```python
from build123d import *

# Parameters (mm, degrees)
VACIADO1_START                    = -69.409306307
VACIADO1_OUTLINE_R                = 22.113173388
VACIADO1_DEPTH                    = 111.965075994
CROQUIS3_W                        = 3
CROQUIS3_H                        = 111.238505794
SALIENTE_EXTRUIR1_DEPTH           = 85
SALIENTE_EXTRUIR1_TAPER           = -0.018
SALIENTE_EXTRUIR1_OTHER_WAY_DEPTH = 2


# Read off the part's stored shape, not the designer's step: Vaciado1
with BuildPart() as part:
    # Croquis1 → Revolución1 (revolve)
    with BuildSketch(Plane.XY, mode=Mode.PRIVATE) as revoluci_n1_sk:
        Polygon((0, 52.555769687), (0, 46.993844398), (0, -69.409306307), (35.29141641, -69.409306307), (35.29141641, -64.244661396), (32.113173388, -64.244661396), (32.113173388, 46.993844398), (35.29141641, 46.993844398), (35.29141641, 52.555769687), align=None)
    revolve(revoluci_n1_sk.sketch.rotate(Axis((0, -77.4814163, 0), (0, 1, 0)), 90), axis=Axis((0, -77.4814163, 0), (0, 1, 0)))

    # Vaciado1 outline → Vaciado1 (cut)
    with BuildSketch(Plane(origin=(0, 0, 0), x_dir=(1, 0, 0), z_dir=(0, 1, 0)).offset(VACIADO1_START)):
        Circle(VACIADO1_OUTLINE_R)
    extrude(amount=VACIADO1_DEPTH, mode=Mode.SUBTRACT)

    # Croquis3 → Saliente-Extruir1 (add)
    with BuildSketch(Plane(origin=(35.21176327, 0, 0), x_dir=(1, 0, 0), z_dir=(0, 0, 1))):
        with Locations((0, -8.625408499)):
            Rectangle(CROQUIS3_W, CROQUIS3_H)
    extrude(amount=-SALIENTE_EXTRUIR1_DEPTH, taper=SALIENTE_EXTRUIR1_TAPER)

    # Croquis3 → Saliente-Extruir1 other way (add)
    with BuildSketch(Plane(origin=(35.21176327, 0, 0), x_dir=(1, 0, 0), z_dir=(0, 0, 1))):
        with Locations((0, -8.625408499)):
            Rectangle(CROQUIS3_W, CROQUIS3_H)
    extrude(amount=SALIENTE_EXTRUIR1_OTHER_WAY_DEPTH)


solid = part.part
```
Could you check a few things on this model? Use its own coordinates, in mm. A direction names the side the tool comes from. Give positions to 0.01 mm unless a question says otherwise; leave off trailing zeros. Order: outer loops, then holes, each group sorted by start corner. A loop starts at its lowest first (then second) coordinate and runs counter-clockwise, first axis right, second up.
Q1. I'm going to push flat-ended pins straight in: P1, Ø8, axis at x = 27, z = -30.5, coming from the +Y side; P2, Ø12, axis at x = -4, y = 37.5, coming from the +Z side; P3, Ø1.2, axis at x = 36.5, z = 1, coming from the -Y side; P4, Ø13.5, axis at x = -2, z = 2.5, coming from the -Y side. Where does each tip first touch, or does it pass through?
Q2. Suppose I cut it at D-D, the plane x = -25. Write out the boundary of the cut face in (y, z), and give its area (3 significant figures).
Q3. Suppose I cut it at B-B, the plane x = 0. Write out the boundary of the cut face in (y, z).
Q4. Suppose I cut it at A-A, the plane y = 37. Count the separate pieces of the cut face and the enclosed holes in it, and give its area (3 significant figures).
Q5. If I drill on line 1 along X through (y, z) = (-19, 0); line 2 along Y through (x, z) = (-25, 22); line 3 along X through (y, z) = (11.5, -66), over which ranges is the centre line in solid material (lowest first)?
Q6. For faces 1 (the cylindrical face through (11.888, -14.211, -18.646)), 2 (the flat face through (-32, -64.245, -8)), 3 (the flat face through (35, -8, 2)), 4 (the flat face through (23, -69.409, 0)), which set-ups out of +Z, -Z, +X, -X, +Y, -Y let a thin tool reach every point of the face, with its end or its side?
Q7. We'd pull the mould along Z, two halves only. Please class faces 5 (the flat face through (0, 52.556, 0)), 6 (the flat face through (0, 42.556, 0)), 7 (the flat face through (35, -9, -85)): +Z half, -Z half, draft (parallel to the pull), parting line (faces both ways), or undercut.
Q8. Suppose I cut it at C-C, the plane x = 19. Write out the boundary of the cut face in (y, z).
Solution:
1. P1: passes through
1. P2: stops at z = 32.11
1. P3: stops at y = -64.24
1. P4: stops at y = 42.56
2. outline: (-69.41, -24.91) - (-64.24, -24.91) - (-64.24, -20.16) - (46.99, -20.16) - (46.99, -24.91) - (52.56, -24.91) - (52.56, 24.91) - (46.99, 24.91) - (46.99, 20.16) - (-64.24, 20.16) - (-64.24, 24.91) - (-69.41, 24.91) - close
2. area: 5,020 mm2
3. outline: (-69.41, -35.29) - (-64.24, -35.29) - (-64.24, -32.11) - (46.99, -32.11) - (46.99, -35.29) - (52.56, -35.29) - (52.56, 35.29) - (46.99, 35.29) - (46.99, 32.11) - (-64.24, 32.11) - (-64.24, 35.29) - (-69.41, 35.29) - (-69.41, 22.11) - (42.56, 22.11) - (42.56, -22.11) - (-69.41, -22.11) - close
4. separate pieces: 2
4. enclosed holes: 1
4. area: 1,970 mm2
5. line 1: x = -32.11 to -22.11, 22.11 to 32.11, 33.71 to 36.71
5. line 2: y = -69.41 to -64.24, 46.99 to 52.56
5. line 3: x = 33.69 to 36.73
6. face 1: -Y
6. face 2: none
6. face 3: +Z, +X
6. face 4: +Z, -Z, +X, -X, -Y
7. face 5: draft
7. face 6: undercut
7. face 7: -Z half
8. outline: (-69.41, -29.74) - (-64.24, -29.74) - (-64.24, -25.89) - (46.99, -25.89) - (46.99, -29.74) - (52.56, -29.74) - (52.56, 29.74) - (46.99, 29.74) - (46.99, 25.89) - (-64.24, 25.89) - (-64.24, 29.74) - (-69.41, 29.74) - (-69.41, 11.31) - (42.56, 11.31) - (42.56, -11.31) - (-69.41, -11.31) - close
